For this review, take the finished solid that the model builds, in its own axes (mm). Face numbers are marked on the shaded views. A direction names the side the tool comes from. Give positions to 0.01 mm unless a question says otherwise; leave off trailing zeros. Loops run counter-clockwise (first coordinate to the right, second up) from the corner with the lowest first, then second, coordinate; pieces in that order, holes last. Notation, with made-up numbers: (45.5, -35) -> (98.5, -35) arc R21 ccw to (98.5, -1) -> close; hole circle Ø1 at (-20, 41.25). An arc over 180 degrees is marked (long way). One line per question, with ' | ' between items. Start each with the question number.
(1) Insertion check: P1, Ø6, axis at x = 73, z = 34, coming from the -Y side; P2, Ø1, axis at y = 12, z = -2.5, coming from the -X side; P3, Ø10, axis at x = 49, y = 7, coming from the +Z side; P4, Ø2, axis at x = 24, y = 16.5, coming from the -Z side. Each pin has a flat end and moves straight along its axis. Give the tip position at first contact, or say it passes through.
(2) Draft analysis for pull direction Z (two halves, no side actions). For the marked faces 4, 5 and 6, state which applies: +Z half, -Z half, draft (parallel to the pull), parting line (faces both ways), or undercut.
(3) Tool access review of the marked faces 1, 2 and 3: name each direction out of +Z, -Z, +X, -X, +Y, -Y from which nothing blocks a thin tool from reaching the whole face with its end or side.
(4) Consider section C-C (x = 0). Write out the cut boundary in (y, z).
(5) Consider section D-D (y = 7.25). Write out the cut boundary in (x, z).
(6) Consider section B-B (z = 76). Write out the cut boundary in (x, y), and give its area (3 significant figures).
(7) Wall thickness on probe 1 along Z at (x, y) = (0, 9); probe 2 along Z at (x, y) = (70, 11.25); probe 3 along X at (y, z) = (9, 40): over which ranges is each line inside the solid? List them lowest first.
(8) Consider section A-A (x = -20). Write out the cut boundary in (y, z), and give its area (3 significant figures).
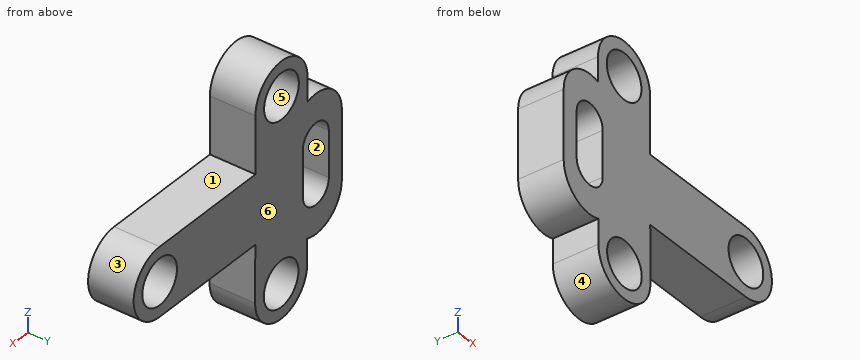
Autodesk Fusion 360 part; units mm, degrees
sketch "Sketch1" plane through (0, 0, 0) normal (0, 1, 0) x (1, 0, 0)
  circle A0 centre (-0.1967, -80) radius 10
  circle A1 centre (-0.1967, -80) radius 5
  circle A2 centre (0, 0) radius 5
  circle A3 centre (0, 0) radius 10
  circle A4 centre (70, -40) radius 10
  circle A5 centre (70, -40) radius 5
  line L0 (-27.5, -30) -> (-27.5, -50)
  arc A6 (-27.5, -50) -> (-12.5, -50) centre (-20, -50) ccw
  line L1 (-12.5, -50) -> (-12.5, -30)
  arc A7 (-12.5, -30) -> (-27.5, -30) centre (-20, -30) ccw
  line L2 (-20, -30) -> (-20, -50) construction
  line L3 (-35, -25) -> (-35, -55)
  arc A8 (-35, -55) -> (-15.168, -69.2004) centre (-20, -55) ccw
  arc A9 (-15.0308, -10.847) -> (-35, -25) centre (-20, -25) ccw
  line L4 (-20, -25) -> (-20, -55) construction
  line L5 (70, -25) -> (14.8802, -25)
  line L6 (70, -55) -> (14.8033, -55)
  line L7 (-15, 0) -> (-15.0308, -10.847)
  line L8 (15, 0) -> (14.8802, -25)
  line L9 (14.8033, -80) -> (14.8033, -55)
  arc A10 (14.9993, -0.1437) -> (-15, 0) centre (0, 0) ccw
  line L10 (-15.1967, -79.96) -> (-15.168, -69.2004)
  arc A11 (-15.1967, -79.96) -> (14.8033, -80) centre (-0.1967, -80) ccw
  arc A12 (70, -55) -> (70, -25) centre (70, -40) ccw
  point P0 (-20, -40)
  point P1 (-20, -40)
  dimension "d1" = 30
  dimension "d2" = 20
  dimension "d3" = 10
  dimension "d4" = 10
  dimension "d5" = 20
  dimension "d6" = 30
  dimension "d7" = 30
  dimension "d8" = 20
  dimension "d9" = 10
  dimension "d10" = 15
  dimension "d11" = 20
  dimension "d12" = 80
  dimension "d13" = 70
  dimension "d14" = 40
  dimension "d15" = 20
  dimension "d16" = 30
  dimension "d17" = 30
  dimension "d18" = 30
extrude "Extrude1" add sketch "Sketch1" along normal blind 20 contours L3 A8 A9 L5 L6 L7 L8 L9 A10 L10 A11 A12
A:
1) P1: passes through | P2: stops at x = -14.87 | P3: stops at z = 55 | P4: stops at z = 25
2) face 4: -Z half | face 5: undercut | face 6: draft
3) face 1: +Z, +X, +Y, -Y | face 2: +Y, -Y | face 3: +X, +Y, -Y
4) outline: (0, -15) -> (20, -15) -> (20, -10) -> (0, -10) -> close; (0, 10) -> (20, 10) -> (20, 70) -> (0, 70) -> close; (0, 90) -> (20, 90) -> (20, 95) -> (0, 95) -> close
5) outline: (-35, 25) arc R15 ccw to (-15.03, 10.85) -> (-15, 0) arc R15 ccw to (15, 0) -> (14.88, 25) -> (70, 25) arc R15 ccw to (70, 55) -> (14.8, 55) -> (14.8, 80) arc R15 ccw to (-15.2, 79.96) -> (-15.17, 69.2) arc R15 ccw to (-35, 55) -> close; hole (-27.5, 30) arc R7.5 ccw to (-12.5, 30) -> (-12.5, 50) arc R7.5 ccw to (-27.5, 50) -> close; hole circle Ø20 at (-0.2, 80); hole circle Ø20 at (0, 0); hole circle Ø20 at (70, 40)
6) outline: (-15.19, 0) -> (-9.36, 0) -> (-9.36, 20) -> (-15.19, 20) -> close; (8.97, 0) -> (14.8, 0) -> (14.8, 20) -> (8.97, 20) -> close | area: 233 mm^2
7) probe 1: z = -15 to -10, 10 to 70, 90 to 95 | probe 2: z = 25 to 30, 50 to 55 | probe 3: x = -35 to -27.5, -12.5 to 60, 80 to 85
8) outline: (0, 10) -> (20, 10) -> (20, 22.5) -> (0, 22.5) -> close; (0, 57.5) -> (20, 57.5) -> (20, 70) -> (0, 70) -> close | area: 500 mm^2
